Work out the finished part from the listing and answer in its coordinate system (mm). Round coordinates to 2 decimals unless told otherwise and drop trailing zeros. Write each loop counter-clockwise with the first axis right and the second up, starting at its lowest first coordinate (ties: lowest second). Pieces come first, ordered by that corner, then holes. Notation, with made-up numbers: (19, 8) - (52, 8) arc R29 ccw to (52, 44) - close; hole circle Ø9 at (70.5, 74). An arc over 180 degrees is marked (long way). Write item = value, one per line. Start each with the question number.
from build123d import *

# Parameters (mm, degrees)
SKETCH1_W           = 1695.45
SKETCH1_H           = 180.975
BOSS_EXTRUDE1_DEPTH = 19.05
SKETCH2_W           = 38.1
SKETCH2_H           = 92.075
BOSS_EXTRUDE3_DEPTH = 19.05
CHAMFER1_SIZE       = 2.54
CHAMFER2_SIZE       = 2.54


with BuildPart() as part:
    # Sketch1 → Boss-Extrude1 (new body)
    with BuildSketch(Plane(origin=(0, 0, 0), x_dir=(1, 0, 0), z_dir=(0, 1, 0))):
        with Locations((847.725, 90.4875)):
            Rectangle(SKETCH1_W, SKETCH1_H)
        with BuildLine():
            Line((254, 118.25605), (312.7502, 118.25605))
            ThreePointArc((312.7502, 118.25605), (325.4502, 105.55605), (312.7502, 92.85605))
            Line((312.7502, 92.85605), (254, 92.85605))
            ThreePointArc((254, 92.85605), (241.3, 105.55605), (254, 118.25605))
        make_face(mode=Mode.SUBTRACT)
    extrude(amount=BOSS_EXTRUDE1_DEPTH)

    # Sketch2 → Boss-Extrude3 (add, through all)
    with BuildSketch(Plane(origin=(0, 19.05, 0), x_dir=(1, 0, 0), z_dir=(0, 1, 0))):
        with Locations((-19.05, 46.0375)):
            Rectangle(SKETCH2_W, SKETCH2_H)
    extrude(amount=-BOSS_EXTRUDE3_DEPTH)

    # Chamfer1
    chamfer1_edges = [part.edges().sort_by_distance(p)[0] for p in [
        (1695.45, 19.05, -90.4875),
        (325.4502, 19.05, -105.55605),
        (847.725, 19.05, -180.975),
        (283.3751, 19.05, -118.25605),
        (241.3, 19.05, -105.55605),
        (283.3751, 19.05, -92.85605),
        (-19.05, 19.05, -92.075),
        (-38.1, 19.05, -46.0375),
        (0, 19.05, -136.525),
        (828.675, 19.05, 0),
    ]]
    chamfer(chamfer1_edges, length=CHAMFER1_SIZE)

    # Chamfer2
    chamfer2_edges = [part.edges().sort_by_distance(p)[0] for p in [
        (325.4502, 0, -105.55605),
        (283.3751, 0, -118.25605),
        (241.3, 0, -105.55605),
        (283.3751, 0, -92.85605),
        (-38.1, 0, -46.0375),
        (-19.05, 0, -92.075),
        (847.725, 0, -180.975),
        (1695.45, 0, -90.4875),
        (828.675, 0, 0),
        (0, 0, -136.525),
    ]]
    chamfer(chamfer2_edges, length=CHAMFER2_SIZE)


solid = part.part
1. Consider line 1 (Z direction, x = 284.5, y = 15.5) (3 decimals); line 2 (X direction, y = 2.5, z = -148.5); line 3 (X direction, y = 16, z = -108). Determine where each line is inside the solid, lowest interval first.
2. Find section A-A on y = 8. Give the vertices of the cut face in (x, z) (3 decimals).
3. This flat-tipped pin is pushed along its axis until it touches: pin 1 (11 mm diameter, centred on y = 12.5, z = -119.5, fed in from -X). Where does it stop, or does it pass through?
Answer key:
q1.line_1 = -180.975 to -118.256, -92.856 to 0
q1.line_2 = 0.04 to 1695.41
q1.line_3 = 0 to 241.54, 325.21 to 1695.45
q2.outline = (-38.1, -92.075) - (0, -92.075) - (0, -180.975) - (1695.45, -180.975) - (1695.45, 0) - (-38.1, 0) - close; hole (254, -118.256) - (312.75, -118.256) arc R12.7 ccw to (312.75, -92.856) - (254, -92.856) arc R12.7 ccw to start
q3.pin_1 = 0
